Check sheet for the modelled part. Datum: model origin and axes. Units: mm. A direction names the side the tool comes from. Round coordinates to 2 decimals unless told otherwise and drop trailing zeros. Loops run counter-clockwise (first coordinate to the right, second up) from the corner with the lowest first, then second, coordinate; pieces in that order, holes last. Notation, with made-up numbers: (-33.75, 20.25) -> (23.25, 20.25) arc R20 cw to (23.25, 41.25) -> close; hole circle Ø10 at (68.25, -31.75). An arc over 180 degrees is marked (long way). Use one line per item in the form item = value. Start each with the question number.
(1) Set-up check for faces 1 (the flat face through (377.825, -20, -9)), 2 (the flat face through (381, -19, -9)): record each of +Z, -Z, +X, -X, +Y, -Y from which the full face is reachable in a straight line by a thin tool's end or side.
(2) Sectioned sample at A-A (y = -19.05). Record the cut outline in (x, z) (1 decimal), and give its area (3 significant figures).
(3) Sectioned sample at C-C (z = -461.5). Record the cut outline in (x, y) (3 decimals), and give its area (3 significant figures).
(4) Sectioned sample at B-B (x = -119). Record the cut outline in (y, z) (3 decimals), and give its area (3 significant figures).
(5) Material ranges on probe 1 along Z at (x, y) = (279.5, -15) (3 decimals); probe 2 along X at (y, z) = (-19, -649); probe 3 along X at (y, z) = (-23, -281.5) (3 decimals), recorded low to high. Write a range as [from, to].
(6) Go/stop test with a flat-tipped pin: pin 1 (8 mm diameter, centred on x = 108.5, z = -33.5, fed in from -Y) (3 decimals). Record where the tip stops, or that it passes through.
(7) Draft check along X on faces 3 (the flat face through (-5, -3.175, 9)), 4 (the flat face through (-381, -19, -9)), 5 (the flat face through (-5, 0, 9)). Enter one of: released by +X, released by -X, zero draft, split by the parting line, or undercut.
from build123d import *

# Parameters (mm, degrees)
F0_W     = 762
F0_H     = 1301.75
F1_DEPTH = 38.1
F2_T     = -3.175
F3_R     = 6.4135
F4_DEPTH = 1301.751


with BuildPart() as f1:
    # F0 (on Front) → F1 (new body)
    with BuildSketch(Plane.XZ):
        Rectangle(F0_W, F0_H)
    extrude(amount=F1_DEPTH)

    # F2
    f2_openings = [f1.faces().sort_by_distance(p)[0] for p in [
        (0, -38.1, 0),
    ]]
    offset(amount=F2_T, openings=f2_openings)

    # F3 (on face) → F4 (cut, through all)
    with BuildSketch(Plane.XY.offset(650.875)):
        with Locations((-285.75, -19.05)):
            Circle(F3_R)
    extrude(amount=-F4_DEPTH, mode=Mode.SUBTRACT)


solid = f1.part
Checks:
q1.face_1 = -Y
q1.face_2 = +Z, -Z, +X, +Y, -Y
q2.outline = (-381, -650.9) -> (-292.2, -650.9) -> (-292.2, -647.7) -> (-377.8, -647.7) -> (-377.8, 647.7) -> (-292.2, 647.7) -> (-292.2, 650.9) -> (-381, 650.9) -> close; (-279.3, -650.9) -> (381, -650.9) -> (381, 650.9) -> (-279.3, 650.9) -> (-279.3, 647.7) -> (377.8, 647.7) -> (377.8, -647.7) -> (-279.3, -647.7) -> close
q2.area = 13,000 mm2
q3.outline = (-381, -38.1) -> (-377.825, -38.1) -> (-377.825, -3.175) -> (377.825, -3.175) -> (377.825, -38.1) -> (381, -38.1) -> (381, 0) -> (-381, 0) -> close
q3.area = 2,640 mm2
q4.outline = (-38.1, -650.875) -> (0, -650.875) -> (0, 650.875) -> (-38.1, 650.875) -> (-38.1, 647.7) -> (-3.175, 647.7) -> (-3.175, -647.7) -> (-38.1, -647.7) -> close
q4.area = 4,350 mm2
q5.probe_1 = [-650.875, -647.7], [647.7, 650.875]
q5.probe_2 = [-381, -292.16], [-279.34, 381]
q5.probe_3 = [-381, -377.825], [377.825, 381]
q6.pin_1 = -3.175
q7.face_3 = undercut
q7.face_4 = released by -X
q7.face_5 = zero draft
